Work out the finished part from the listing and answer in its coordinate system (mm). A direction names the side the tool comes from. Give positions to 0.01 mm unless a question says otherwise; leave off trailing zeros. Loops run counter-clockwise (first coordinate to the right, second up) from the corner with the lowest first, then second, coordinate; pieces in that order, holes last. Notation, with made-up numbers: M 33.5,87.5 L 72.5,87.5 A16 ccw 72.5,95.5 Z; hole C 11.25,81.5 d7. An arc over 180 degrees is marked long. Use a Markdown table: item, result.
Autodesk Inventor part; units mm, degrees
ref_plane "YZ Plane" through (0, 0, 0) normal (1, 0, 0) x (0, 1, 0)
ref_plane "XZ Plane" through (0, 0, 0) normal (0, 1, 0) x (-1, 0, 0)
ref_plane "XY Plane" through (0, 0, 0) normal (0, 0, 1) x (1, 0, 0)
sketch "Sketch1" plane through (0, 0, 0) normal (0, 0, 1) x (1, 0, 0)
  line L0 (0, 0) -> (609.6, 0) construction
  line L1 (609.6, 0) -> (609.6, 209.55)
  line L2 (609.6, 209.55) -> (0, 209.55) construction
  line L3 (0, 209.55) -> (0, 0) construction
  line L4 (0, 0) -> (304.8, 0) construction
  line L5 (304.8, 0) -> (304.8, 165.1) construction
  line L6 (304.8, 165.1) -> (0, 165.1) construction
  line L7 (0, 165.1) -> (0, 0) construction
  line L8 (0, 0) -> (165.1, 0) construction
  line L9 (165.1, 0) -> (165.1, 304.8) construction
  line L10 (165.1, 304.8) -> (0, 304.8) construction
  line L11 (0, 304.8) -> (0, 0) construction
  line L12 (0, 0) -> (177.8, 0) construction
  line L13 (177.8, 0) -> (177.8, 177.8) construction
  line L14 (177.8, 177.8) -> (0, 177.8) construction
  line L15 (0, 177.8) -> (0, 0) construction
  circle A0 centre (177.8, 177.8) radius 12.7
  line L16 (177.8, 177.8) -> (165.1, 177.8)
  line L17 (177.8, 177.8) -> (177.8, 165.1)
  line L18 (177.8, 177.8) -> (168.819744, 168.819744)
  line L19 (177.8, 177.8) -> (190.5, 177.8) construction
  line L20 (168.819744, 168.819744) -> (52.076414, 52.076414) construction
  line L21 (168.819744, 168.819744) -> (333.919744, 168.819744) construction
  line L22 (177.8, 165.1) -> (177.8, 0) construction
  line L23 (165.1, 177.8) -> (0, 177.8) construction
  arc A1 (0, 177.8) -> (177.8, 0) centre (177.8, 177.8) ccw
  line L24 (177.8, 177.8) -> (355.6, 177.8) construction
  line L25 (355.6, 177.8) -> (355.6, 193.675)
  line L26 (355.6, 193.675) -> (177.8, 193.675) construction
  line L27 (177.8, 193.675) -> (177.8, 177.8) construction
  circle A2 centre (355.6, 193.675) radius 12.7
  line L28 (355.6, 193.675) -> (482.6, 193.675) construction
  line L29 (482.6, 193.675) -> (482.6, 209.55) construction
  line L30 (482.6, 209.55) -> (355.6, 209.55) construction
  line L31 (355.6, 209.55) -> (355.6, 193.675) construction
  circle A3 centre (482.6, 209.55) radius 12.7
  line L32 (177.8, 0) -> (609.6, 0)
  line L33 (177.8, 165.1) -> (355.6, 180.975)
  line L34 (482.6, 196.85) -> (355.6, 180.975)
  line L35 (482.6, 196.85) -> (609.6, 209.55)
  line L36 (165.1, 177.8) -> (165.1, 304.8) construction
  line L37 (165.1, 304.8) -> (241.3, 304.8) construction
  circle A4 centre (241.3, 304.8) radius 76.2
  circle A5 centre (177.8, 228.6) radius 12.7
  line L38 (177.8, 177.8) -> (177.8, 228.6)
  line L39 (0, 177.8) -> (0, 304.8)
  line L40 (241.3, 304.8) -> (195.441695, 365.656026) construction
  line L41 (241.3, 304.8) -> (317.5, 304.8) construction
  line L42 (195.441695, 365.656026) -> (354.191695, 365.656026) construction
  line L43 (195.441695, 365.656026) -> (99.90356, 492.439413) construction
  line L44 (195.441695, 365.656026) -> (354.191695, 365.656026) construction
  line L45 (165.1, 304.8) -> (0, 304.8) construction
  line L46 (241.3, 304.8) -> (169.695422, 330.861935) construction
  line L47 (241.3, 304.8) -> (317.5, 304.8) construction
  line L48 (169.695422, 330.861935) -> (20.519219, 385.157633) construction
  line L49 (177.8, 0) -> (408.09644, 0) construction
  line L50 (241.3, 304.8) -> (317.5, 304.8) construction
  line L51 (241.3, 304.8) -> (175.308864, 342.9) construction
  line L52 (241.3, 304.8) -> (317.5, 304.8) construction
  line L53 (175.308864, 342.9) -> (37.827331, 422.275) construction
  arc A6 (99.90356, 492.439413) -> (20.519219, 385.157633) centre (241.3, 304.8) ccw
  arc A7 (37.827331, 422.275) -> (0, 304.8) centre (330.4977, 263.206429) ccw
  line L54 (37.827331, 422.275) -> (26.828809, 428.625) construction
  circle A8 centre (26.828809, 428.625) radius 12.7
  line L55 (0, 304.8) -> (-12.7, 304.8) construction
  circle A9 centre (-12.7, 304.8) radius 12.7
  line L56 (0, 177.8) -> (-12.7, 177.8) construction
  circle A10 centre (-12.7, 177.8) radius 12.7
  line L57 (52.076414, 52.076414) -> (43.096158, 43.096158) construction
  circle A11 centre (43.096158, 43.096158) radius 12.7
  line L58 (0, 177.8) -> (0, 304.8)
  circle A12 centre (43.096158, 43.096158) radius 11.1125
  circle A13 centre (-12.7, 304.8) radius 11.1125
  circle A14 centre (-12.7, 177.8) radius 11.1125
  circle A15 centre (26.828809, 428.625) radius 11.1125
  line L59 (190.5, 177.8) -> (393.7, 177.8) construction
  line L60 (609.6, 0) -> (-38.1, 0)
  line L61 (-38.1, 0) -> (-38.1, 508)
  line L62 (177.8, 0) -> (-38.1, 0)
  line L63 (-38.1, 508) -> (112.468391, 501.618568)
  line L64 (112.468391, 501.618568) -> (99.90356, 492.439413)
  line L65 (112.468391, 501.618568) -> (-38.1, 501.618568)
  line L66 (-38.1, 501.618568) -> (-38.1, 508)
  line L67 (-38.1, 508) -> (112.468391, 508)
  line L68 (112.468391, 508) -> (112.468391, 501.618568)
  point P0 (165.275068, 230.701449)
  point P1 (172.715134, 216.962383)
  dimension "d16" = 25.4
  dimension "d19" = 25.4
  dimension "d0" = 609.6
  dimension "d1" = 209.55
  dimension "d2" = 304.8
  dimension "d3" = 165.1
  dimension "d4" = 165.1
  dimension "d5" = 304.8
  dimension "d6" = 177.8
  dimension "d7" = 177.8
  dimension "d8" = 25.4
  dimension "d9" = 12.7
  dimension "d10" = 135
  dimension "d11" = 165.1
  dimension "d12" = 135
  dimension "d13" = 165.1
  dimension "d14" = 177.8
  dimension "d15" = 15.875
  dimension "d17" = 127
  dimension "d18" = 15.875
  dimension "d20" = 127
  dimension "d21" = 76.2
  dimension "d22" = 152.4
  dimension "d23" = 25.4
  dimension "d24" = 50.8
  dimension "d25" = 127
  dimension "d26" = 127
  dimension "d33" = 158.75
  dimension "d34" = 127
  dimension "d35" = 160
  dimension "d36" = 158.75
  dimension "d37" = 180
  dimension "d45" = 150
  dimension "d46" = 158.75
  dimension "d47" = 180
  dimension "d48" = 12.7
  dimension "d49" = 12.7
  dimension "d50" = 12.7
  dimension "d52" = 12.7
  dimension "d53" = 25.4
  dimension "d55" = 214.47119
  dimension "d56" = 22.225
  dimension "d57" = 22.225
  dimension "d58" = 22.225
  dimension "d59" = 22.225
  dimension "d60" = 134.70384
  dimension "d72" = 647.7
  dimension "d73" = 508
  dimension "d74" = 90
  dimension "d77" = 150.70356
  dimension "d78" = 15.56059
sketch "Sketch1 outline for Extrusion3" plane through (0, 0, 0) normal (0, 0, 1) x (1, 0, 0)
  line L0 (-38.1, 508) -> (-38.1, 0)
  line L1 (112.468391, 508) -> (-38.1, 508)
  line L2 (112.468391, 501.618568) -> (112.468391, 508)
  line L3 (99.90356, 492.439413) -> (112.468391, 501.618568)
  arc A0 (37.827331, 422.275) -> (99.90356, 492.439413) centre (241.3, 304.8) cw
  arc A1 (20.519219, 385.157633) -> (37.827331, 422.275) centre (241.3, 304.8) cw
  arc A2 (0, 304.8) -> (20.519219, 385.157633) centre (330.4977, 263.206429) cw
  line L4 (0, 177.8) -> (0, 304.8)
  arc A3 (52.076414, 52.076414) -> (0, 177.8) centre (177.8, 177.8) cw
  arc A4 (177.8, 0) -> (52.076414, 52.076414) centre (177.8, 177.8) cw
  line L5 (-38.1, 0) -> (177.8, 0)
  circle A5 centre (-12.7, 177.8) radius 12.7
  arc A6 (52.076414, 52.076414) -> (55.796158, 43.096158) centre (43.096158, 43.096158) ccw
  arc A7 (55.796158, 43.096158) -> (52.076414, 52.076414) centre (43.096158, 43.096158) ccw
  circle A8 centre (-12.7, 304.8) radius 12.7
  arc A9 (37.827331, 422.275) -> (39.528809, 428.625) centre (26.828809, 428.625) ccw
  arc A10 (39.528809, 428.625) -> (37.827331, 422.275) centre (26.828809, 428.625) ccw
extrude "Extrusion3" add sketch "Sketch1 outline for Extrusion3" along normal blind 25.4
(1) Given P1, Ø3, axis at y = 504.5, z = 19, coming from the +X side; P2, Ø8, axis at y = 82.5, z = 3.5, coming from the +X side; P3, Ø7.5, axis at y = 247, z = 7, coming from the +X side, each flat-ended and moving along its own axis, determine where each tip first touches the part or whether it passes through.
Entries:
| item | result |
|---|---|
| P1 | stops at x = 112.47 |
| P2 | stops at x = 30.31 |
| P3 | stops at x = 0 |
(2) A cutting plane is placed at A-A (x = -12.7). Write down the section's boundary in (y, z), and give its area (3 significant figures).
Entries:
| item | result |
|---|---|
| outline | M 0,0 L 165.1,0 L 165.1,25.4 L 0,25.4 Z; M 190.5,0 L 292.1,0 L 292.1,25.4 L 190.5,25.4 Z; M 317.5,0 L 508,0 L 508,25.4 L 317.5,25.4 Z |
| area | 11,600 mm² |
(3) A cutting plane is placed at C-C (y = 222). Write down the section's boundary in (x, z), and give its area (3 significant figures).
Entries:
| item | result |
|---|---|
| outline | M -38.1,0 L 0,0 L 0,25.4 L -38.1,25.4 Z |
| area | 968 mm² |
(4) Which of the six approach directions +Z, -Z, +X, -X, +Y, -Y give full straight-line access (tool end or side, diameter ignored) to faces 1 (the cylindrical face through (13.91, 108.86, 12.52)), 2 (the flat face through (-3, 274, 0))?
Entries:
| item | result |
|---|---|
| face 1 | +Z, -Z, +X |
| face 2 | -Z, +X, -X, +Y, -Y |
(5) Consider probe 1 along Y at (x, z) = (-12.7, 8); probe 2 along Y at (x, z) = (-3.5, 8.75) (3 decimals); probe 3 along Y at (x, z) = (38.5, 22.5). Determine where each line is inside the solid, lowest interval first. Write a range as [from, to].
Entries:
| item | result |
|---|---|
| probe 1 | y = [0, 165.1], [190.5, 292.1], [317.5, 508] |
| probe 2 | y = [0, 169.045], [186.555, 296.045], [313.555, 508] |
| probe 3 | y = [0, 31.26], [54.94, 67.31], [423.43, 423.62], [433.63, 508] |
(6) A cutting plane is placed at D-D (x = 149). Write down the section's boundary in (y, z).
Entries:
| item | result |
|---|---|
| outline | M 0,0 L 2.35,0 L 2.35,25.4 L 0,25.4 Z |
(7) The mould has two halves that part along Y. Classify faces 3 (the flat face through (-3, 274, 25.4)), 4 (the cylindrical face through (110.663, 13.163, 12.522)), 5 (the flat face through (68, 0, 13)): released by +Y, released by -Y, zero draft, split by the parting line, or undercut.
Entries:
| item | result |
|---|---|
| face 3 | zero draft |
| face 4 | undercut |
| face 5 | released by -Y |
